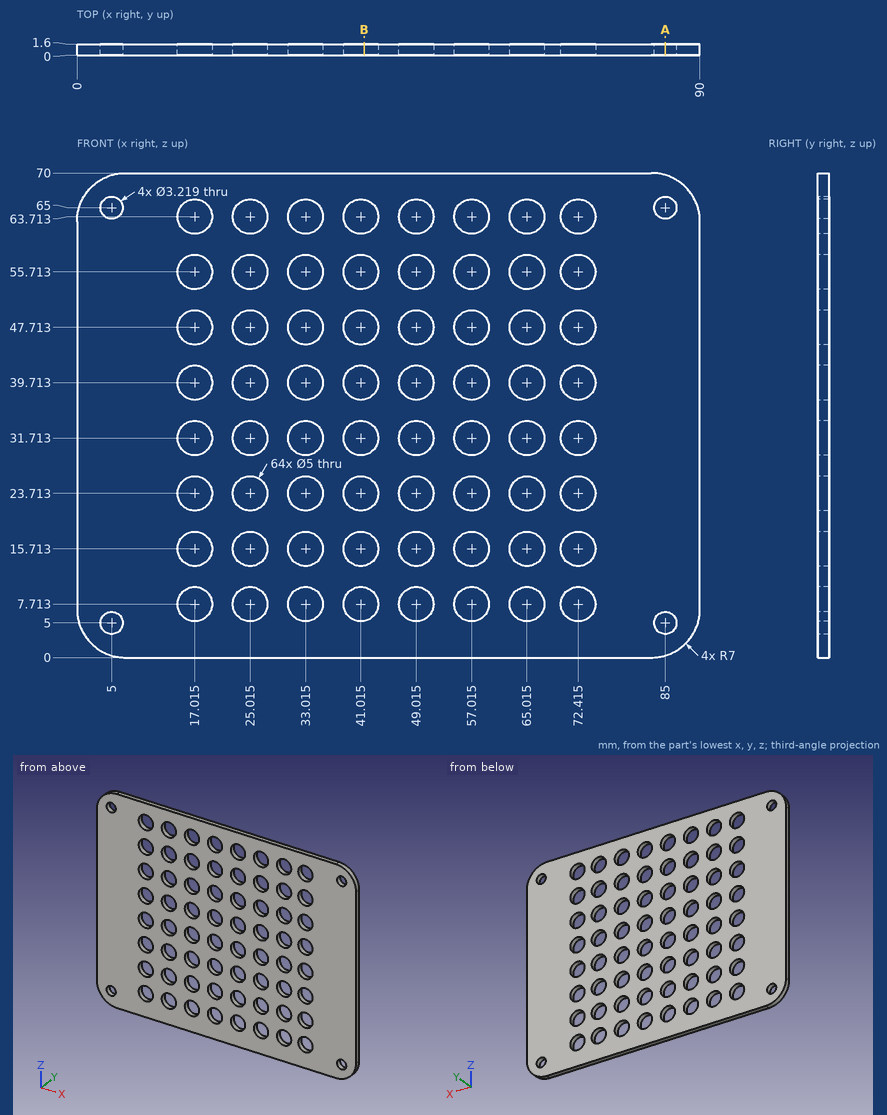
Study the drawing (mm; zero at the part's minimum x, y, z) and answer. Give positions to 0.01 mm unless a question says otherwise; leave off trailing zeros. Write each loop counter-clockwise with the first axis right and the second up, starting at its lowest first coordinate (ties: lowest second). Pieces come first, ordered by that corner, then holes.
(1) A straight line is drawn through the part: line 1 (Z direction, x = 5, y = 0.7). Find the intervals that lie inside material, in ascending order.
Final values:
line 1: z = 0.29 to 3.39, 6.61 to 63.39, 66.61 to 69.71
(2) The part is cut by section B-B on x = 41.5. Count the separate pieces of the cut face and the enclosed holes in it.
Final values:
separate pieces: 9
enclosed holes: 0
(3) The part is cut by section A-A on x = 85. Write down the section's boundary in (y, z), plus the area to 3 significant figures.
Final values:
outline: (0, 0.29) - (1.6, 0.29) - (1.6, 3.39) - (0, 3.39) - close; (0, 6.61) - (1.6, 6.61) - (1.6, 63.39) - (0, 63.39) - close; (0, 66.61) - (1.6, 66.61) - (1.6, 69.71) - (0, 69.71) - close
area: 101 mm2
